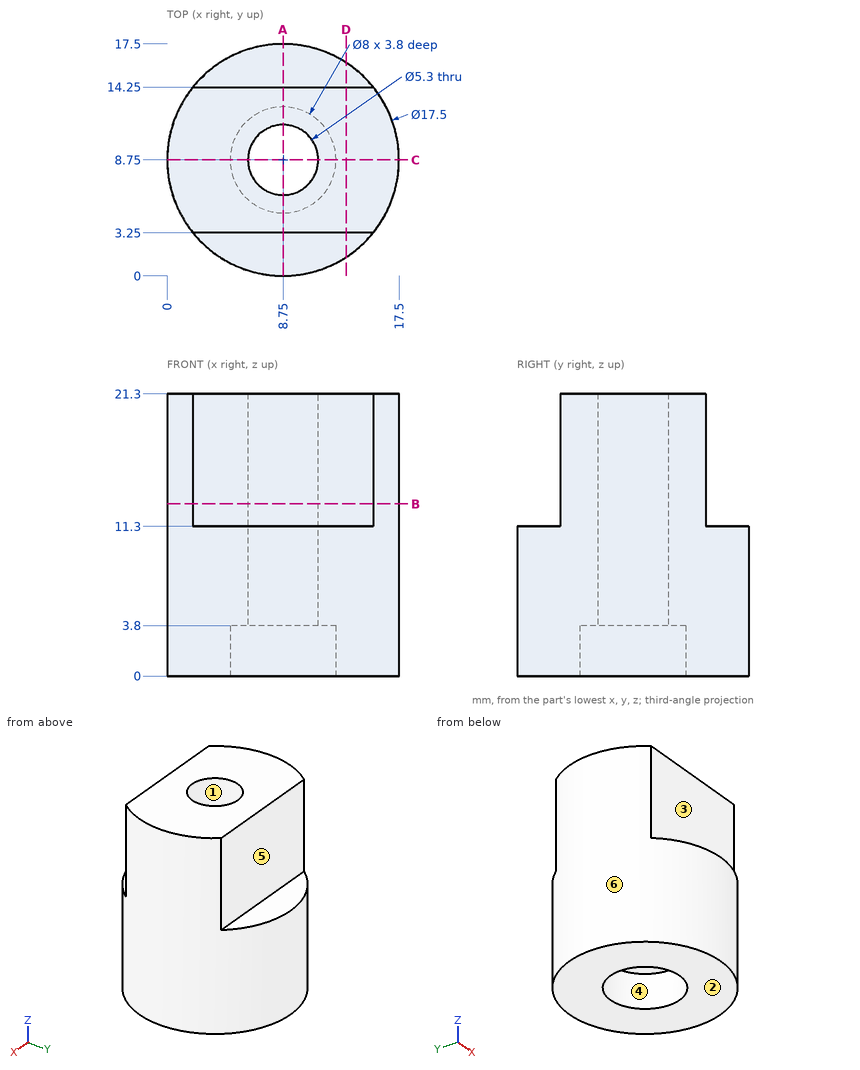
Can you work these out from the drawing? Everything is in mm from the part's minimum corner. A direction names the side the tool comes from. Round coordinates to 2 decimals unless told otherwise and drop trailing zeros. Order: outer loops, then holes, each group sorted by start corner. A loop starts at its lowest first (then second) coordinate and runs counter-clockwise, first axis right, second up. Notation, with made-up numbers: (15.5, -13) - (33.5, -13) arc R28 cw to (33.5, 21) - close; hole circle Ø3 at (41.5, 69). An arc over 180 degrees is marked (long way). Answer in a Markdown table with one row per item.
(1) Suppose I cut it at D-D, the plane x = 13.5. Please give me the cut outline in (y, z).
From the geometry:
| item | result |
|---|---|
| outline | (1.4, 0) - (16.1, 0) - (16.1, 11.3) - (14.25, 11.3) - (14.25, 21.3) - (3.25, 21.3) - (3.25, 11.3) - (1.4, 11.3) - close |
(2) Which directions (+Z, -Z, +X, -X, +Y, -Y) give clear straight access to the entire face, cutting with the end or side of a thin tool? Please do the marked faces 4, 5 and 6.
From the geometry:
| item | result |
|---|---|
| face 4 | -Z |
| face 5 | +Z, +X, -X, +Y |
| face 6 | +Z, -Z |
(3) Suppose I cut it at A-A, the plane x = 8.75. Please give me the cut outline in (y, z).
From the geometry:
| item | result |
|---|---|
| outline | (0, 0) - (4.75, 0) - (4.75, 3.8) - (6.1, 3.8) - (6.1, 21.3) - (3.25, 21.3) - (3.25, 11.3) - (0, 11.3) - close; (11.4, 3.8) - (12.75, 3.8) - (12.75, 0) - (17.5, 0) - (17.5, 11.3) - (14.25, 11.3) - (14.25, 21.3) - (11.4, 21.3) - close |
(4) Please list where these lines run through material, in increasing order: L1, parallel to Y at x = 8.75, z = 10.5; L2, parallel to Y at x = 14, z = 13.75; L3, parallel to Y at x = 8.75, z = 2.75. Write a range as from..to.
From the geometry:
| item | result |
|---|---|
| L1 | y = 0..6.1, 11.4..17.5 |
| L2 | y = 3.25..14.25 |
| L3 | y = 0..4.75, 12.75..17.5 |
(5) If we mould it in two halves opening along Y, with no side actions, what happens to the marked faces 1, 2 and 3? For each: released by +Y, released by -Y, zero draft, split by the parting line, or undercut.
From the geometry:
| item | result |
|---|---|
| face 1 | undercut |
| face 2 | zero draft |
| face 3 | released by -Y |
(6) Suppose I cut it at C-C, the plane y = 8.75. Please give me the cut outline in (x, z), plus the area to 3 significant figures.
From the geometry:
| item | result |
|---|---|
| outline | (0, 0) - (4.75, 0) - (4.75, 3.8) - (6.1, 3.8) - (6.1, 21.3) - (0, 21.3) - close; (11.4, 3.8) - (12.75, 3.8) - (12.75, 0) - (17.5, 0) - (17.5, 21.3) - (11.4, 21.3) - close |
| area | 250 mm2 |
(7) For P1, Ø5, axis at x = 7, z = 14.5, coming from the +Y side; P2, Ø2, axis at x = 9.5, y = 6, coming from the -Z side; P3, Ø8, axis at y = 8, z = 9.5, coming from the -X side; P4, Ø4, axis at y = 3.5, z = 17.5, coming from the -X side, each with a flat end and sliding along its axis, tell me the tip position at first contact or that it passes through.
From the geometry:
| item | result |
|---|---|
| P1 | stops at y = 14.25 |
| P2 | stops at z = 3.8 |
| P3 | stops at x = 0 |
| P4 | stops at x = 0.63 |
(8) Suppose I cut it at B-B, the plane z = 13. Please give me the cut outline in (x, y).
From the geometry:
| item | result |
|---|---|
| outline | (1.94, 3.25) - (15.56, 3.25) arc R8.75 ccw to (15.56, 14.25) - (1.94, 14.25) arc R8.75 ccw to start; hole circle Ø5.3 at (8.75, 8.75) |
